Autodesk Inventor part; units mm, degrees
ref_plane "YZ Plane" through (0, 0, 0) normal (1, 0, 0) x (0, 1, 0)
ref_plane "XZ Plane" through (0, 0, 0) normal (0, 1, 0) x (-1, 0, 0)
ref_plane "XY Plane" through (0, 0, 0) normal (0, 0, 1) x (1, 0, 0)
sketch "Sketch1" plane through (0, 0, 0) normal (0, 0, 1) x (1, 0, 0)
  line L0 (0, 0) -> (0, 33)
  line L1 (0, 33) -> (-50, 33)
  line L2 (0, 0) -> (-41.75, 0)
  line L3 (-41.75, 0) -> (-41.75, 5)
  line L4 (-41.75, 5) -> (-39.5, 5)
  line L5 (-39.5, 5) -> (-39.5, 8.7)
  line L6 (-39.5, 8.7) -> (-41.75, 8.7)
  line L7 (-41.75, 8.7) -> (-26.5, 8.7) construction
  line L8 (-41.75, 8.7) -> (-41.75, 27)
  line L9 (-41.75, 27) -> (-50, 27)
  arc A0 (-50, 28.5) -> (-50, 31.5) centre (-50, 30) ccw
  line L10 (-50, 33) -> (-50, 31.5)
  line L11 (-50, 28.5) -> (-50, 27)
  point P0 (-50, 32.25)
  dimension "d0" = 33
  dimension "d1" = 50
  dimension "d2" = 6
  dimension "d3" = 41.75
  dimension "d4" = 5
  dimension "d5" = 3.7
  dimension "d9" = 39.5
  dimension "d65" = 3
  dimension "d66" = 1.5
  dimension "d67" = 8.25
revolve "Revolution1" add sketch "Sketch1" angle 360 about axis through (0, 0, 0) along (0, 1, 0)
sketch "Sketch3" plane through (0, 33, 0) normal (0, 1, 0) x (1, 0, 0)
  circle A0 centre (0, 0) radius 41
  circle A1 centre (0, 23) radius 16.5 construction
  dimension "d17" = 33
  dimension "d25" = 23
hole "Hole1" at (0, 33, -23) direction (0, -1, 0) diameter 30 end through all
sketch "Sketch4" plane through (0, 33, 0) normal (0, 1, 0) x (1, 0, 0)
  circle A0 centre (0, 0) radius 39.5
  point P0 (0, -29)
  dimension "d27" = 29
hole "Hole2" at (0, 33, 29) direction (0, -1, 0) diameter 18 end through all
sketch "Sketch5" plane through (0, 0, 0) normal (1, 0, 0) x (0, 1, 0)
  line L0 (0, 0) -> (0, 5.05)
  line L1 (0, -41.75) -> (0, 41.75)
  line L2 (0, 5.05) -> (3, 5.05)
  line L3 (3, 5.05) -> (3, -5.05)
  line L4 (3, -5.05) -> (0, -5.05)
  line L5 (0, -5.05) -> (0, 0)
  dimension "d35" = 5.05
  dimension "d36" = 3
  dimension "d37" = 10.1
extrude "Extrusion2" cut sketch "Sketch5" against normal through all both and the other way through all
sketch "Sketch6" plane through (0, 33, 0) normal (0, 1, 0) x (1, 0, 0)
  circle A0 centre (0, 23) radius 15
  point P0 (0, 0)
  point P1 (0, 0)
hole "Hole3" at (0, 33, 0) direction (0, -1, 0) diameter 5 end through all
hole "Hole4" at (0, 33, 0) direction (0, -1, 0) diameter 8 depth 20 tip angle 118
sketch "Sketch7" plane through (0, 33, 0) normal (0, 1, 0) x (1, 0, 0)
  circle A0 centre (0, -29) radius 9
  circle A1 centre (0, -29) radius 12
  circle A2 centre (0, 23) radius 15
  circle A3 centre (0, 23) radius 17.5
  point P0 (0, 0)
  dimension "d57" = 24
  dimension "d58" = 35
extrude "Extrusion3" cut sketch "Sketch7" against normal blind 3 contours A0 | A1 | A2 | A3
thread "Thread1"
thread "Thread2"
properties part number "Body glass top" material "Polypropylene"
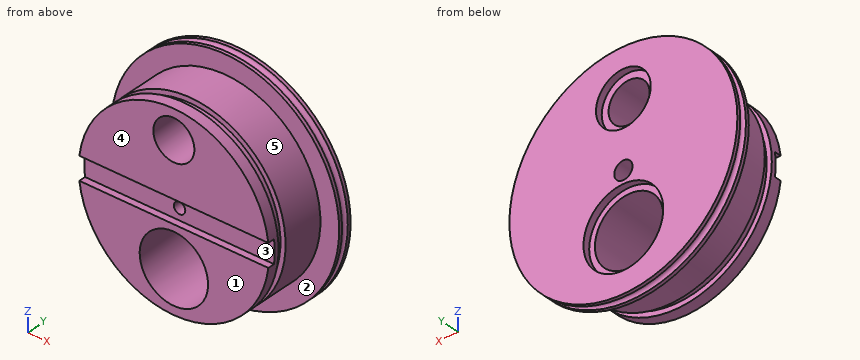
Can you work these out from the model? Positions are in its coordinate system, mm. Face numbers are marked on the shaded views. A direction names the side the tool comes from. Give positions to 0.01 mm unless a question says otherwise; leave off trailing zeros. Loops run counter-clockwise (first coordinate to the right, second up) from the corner with the lowest first, then second, coordinate; pieces in that order, holes last. Notation, with made-up numbers: M 68.5,69 L 85.5,69 A17 ccw 85.5,73 Z; hole C -2,36 d9. An arc over 180 degrees is marked long. One line per item, written item: value.
(1) Will these pins go through, and if not, where does the flat tip stop? pin 1 (20.5 mm diameter, centred on x = 0, z = 29, fed in from +Y); pin 2 (3.5 mm diameter, centred on x = 20.5, y = 1.5, fed in from +Z); pin 3 (10 mm diameter, centred on x = 25, y = 25.5, fed in from +Z); pin 4 (3 mm diameter, centred on x = 0, z = 0, fed in from -Y).
Returned:
pin 1: y = 30
pin 2: z = 37.3
pin 3: z = 45.72
pin 4: through
(2) Which directions (+Z, -Z, +X, -X, +Y, -Y) give clear straight access to the entire face, cutting with the end or side of a thin tool? Please do the marked faces 1 and 2.
Returned:
face 1: +Z, -Z, +X, -X, -Y
face 2: -Y
(3) I need wall thicknesses on line 1 (Z direction, x = 0, y = 17); line 2 (Z direction, x = 0, y = 12); line 3 (Z direction, x = -6, y = 8). Which ranges of each line are inside material? Lowest first, please.
Returned:
line 1: -41.75 to -38, -8 to -4, 4 to 20, 38 to 41.75
line 2: -41.75 to -38, -8 to -2.5, 2.5 to 20, 38 to 41.75
line 3: -39.04 to -36.75, -9.25 to 22.29, 35.71 to 39.04
(4) Suppose I cut it at A-A on z = 0. List the corners of the cut face in (x, y) for me.
Returned:
outline: M -50,27 L -41.75,27 L -41.75,8.7 L -39.5,8.7 L -39.5,5 L -41.75,5 L -41.75,3 L -2.5,3 L -2.5,12.1 L -4,13 L -4,33 L -50,33 L -50,31.5 A1.5 cw -50,28.5 Z; M 2.5,3 L 41.75,3 L 41.75,5 L 39.5,5 L 39.5,8.7 L 41.75,8.7 L 41.75,27 L 50,27 L 50,28.5 A1.5 cw 50,31.5 L 50,33 L 4,33 L 4,13 L 2.5,12.1 Z
(5) We'd pull the mould along Z, two halves only. Please class the marked faces 3, 4 and 5: released by +Z, released by -Z, zero draft, split by the parting line, or undercut.
Returned:
face 3: undercut
face 4: zero draft
face 5: split by the parting line
(6) Suppose I cut it at B-B on x = 0. Count the separate pieces of the cut face and the enclosed holes in it, plus the area to 3 significant figures.
Returned:
separate pieces: 4
enclosed holes: 0
area: 972 mm^2
